The figure shows three views and two pictorial views of one solid part (mm, origin at its lowest corner). Answer the questions. A direction names the side the tool comes from. Give positions to 0.01 mm unless a question says otherwise; leave off trailing zeros. Order: outer loops, then holes, each group sorted by start corner. A loop starts at its lowest first (then second) coordinate and runs counter-clockwise, first axis right, second up. Notation, with made-up numbers: (37.5, -24.75) - (87.5, -24.75) arc R9 cw to (87.5, -16.75) - close; hole circle Ø11 at (-12, -19). An arc over 180 degrees is marked (long way). Write item = value, one per line.
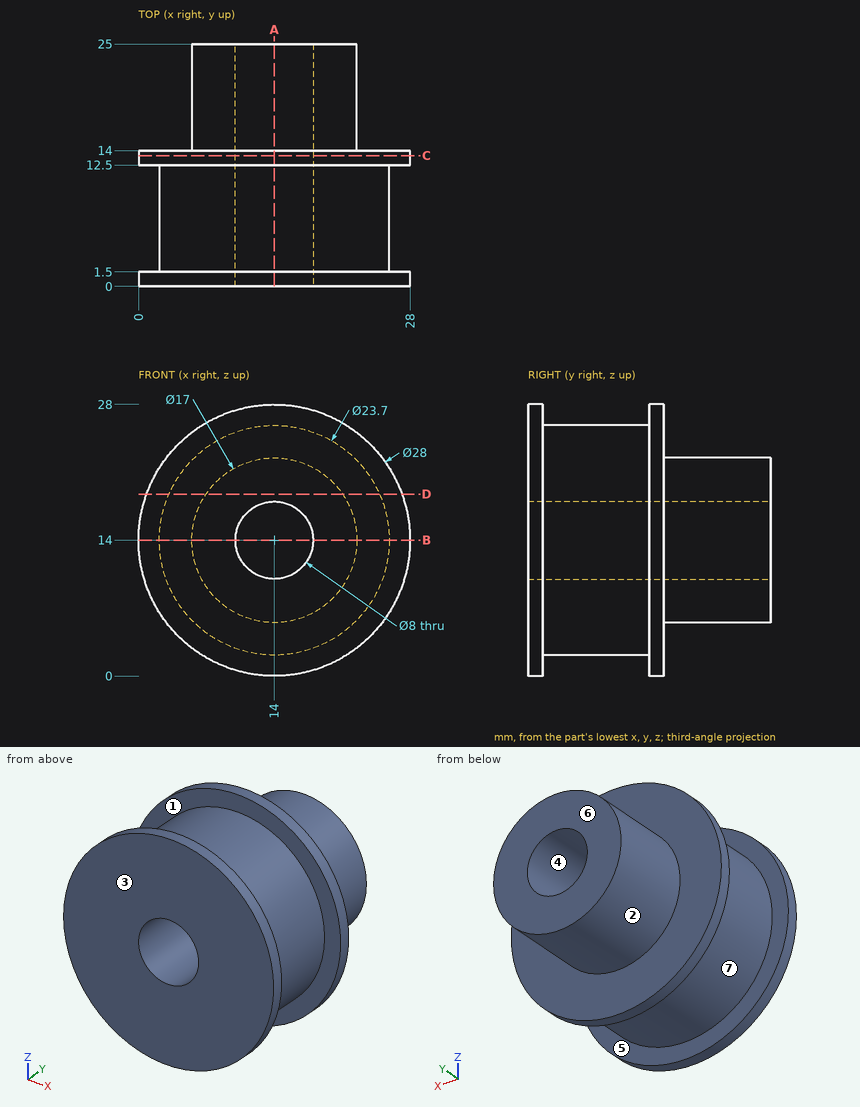
1. Section D-D (z = 18.75) is taken. Determine the outline of the cut face in (x, y), and give its area (3 significant figures).
Recorded:
outline = (0.83, 0) - (27.17, 0) - (27.17, 1.5) - (24.86, 1.5) - (24.86, 12.5) - (27.17, 12.5) - (27.17, 14) - (21.05, 14) - (21.05, 25) - (6.95, 25) - (6.95, 14) - (0.83, 14) - (0.83, 12.5) - (3.14, 12.5) - (3.14, 1.5) - (0.83, 1.5) - close
area = 473 mm^2
2. Section C-C (y = 13.5) is taken. Determine the outline of the cut face in (x, z), and give its area (3 significant figures).
Recorded:
outline = circle Ø28 at (14, 14); hole circle Ø8 at (14, 14)
area = 565 mm^2
3. Section A-A (x = 14) is taken. Determine the outline of the cut face in (y, z), and give its area (3 significant figures).
Recorded:
outline = (0, 0) - (1.5, 0) - (1.5, 2.15) - (12.5, 2.15) - (12.5, 0) - (14, 0) - (14, 5.5) - (25, 5.5) - (25, 10) - (0, 10) - close; (0, 18) - (25, 18) - (25, 22.5) - (14, 22.5) - (14, 28) - (12.5, 28) - (12.5, 25.85) - (1.5, 25.85) - (1.5, 28) - (0, 28) - close
area = 332 mm^2
4. Determine the mould class of the marked faces 4, 5, 6 and 7 for opening direction Y: +Y half, -Y half, draft (parallel to the pull), parting line (faces both ways), or undercut.
Recorded:
face_4 = draft
face_5 = undercut
face_6 = +Y half
face_7 = undercut
5. Flat-ended cylindrical pins translate along their axes: pin 1 (5 mm diameter, centred on y = 9, z = 22.5, fed in from +X); pin 2 (3 mm diameter, centred on x = 9.5, y = 16, fed in from +Z); pin 3 (5 mm diameter, centred on x = 18.5, y = 12, fed in from +Z). Find the tip coordinate at first contact, or state that the pin passes through.
Recorded:
pin_1 = 24.22
pin_2 = 21.95
pin_3 = 27.85
6. For the marked faces 1, 2 and 3, determine the directions among +Z, -Z, +X, -X, +Y, -Y from which every point of the face is accessible in a straight line to the end or side of a thin tool.
Recorded:
face_1 = none
face_2 = +Y
face_3 = +Z, -Z, +X, -X, -Y
7. Straight lines are drawn through the part: L1, parallel to Z at x = 14, y = 8.25; L2, parallel to Y at x = 23.75, z = 4.75; L3, parallel to X at y = 14.75, z = 14. For each, find the intervals that lie inside material, in ascending order. Write a range as [from, to].
Recorded:
L1 = [2.15, 10], [18, 25.85]
L2 = [0, 1.5], [12.5, 14]
L3 = [5.5, 10], [18, 22.5]
8. Section B-B (z = 14) is taken. Determine the outline of the cut face in (x, y).
Recorded:
outline = (0, 0) - (10, 0) - (10, 25) - (5.5, 25) - (5.5, 14) - (0, 14) - (0, 12.5) - (2.15, 12.5) - (2.15, 1.5) - (0, 1.5) - close; (18, 0) - (28, 0) - (28, 1.5) - (25.85, 1.5) - (25.85, 12.5) - (28, 12.5) - (28, 14) - (22.5, 14) - (22.5, 25) - (18, 25) - close
